Part model, mm, in its own coordinate system. Face numbers are marked on the shaded views. A direction names the side the tool comes from. Coordinates: 2 decimals unless noted, no trailing zeros. Order: outer loops, then holes, each group sorted by start corner. A loop starts at its lowest first (then second) coordinate and runs counter-clockwise, first axis right, second up.
1) Tool access for the marked faces 4, 5, 6 and 7: list every direction of +Z, -Z, +X, -X, +Y, -Y with a clear straight run to the whole face (end or side of a thin tool).
2) Wall check: L1, parallel to Z at x = -22, y = -8; L2, parallel to X at y = -13.5, z = 18.5; L3, parallel to X at y = -8.75, z = 11. Give the ranges that are in metal, low to high.
3) Cut at C-C (y = -8.5). List the corners of the cut face in (x, z).
4) Cut at B-B (z = 23). List the corners of the cut face in (x, y), and give its area (3 significant figures).
5) Cut at A-A (x = -9). List the corners of the cut face in (y, z).
6) Pin check, flat tips, straight feed: pin 1 Ø2 at (x, y) = (17, -13) entering from -Z; pin 2 Ø1 at (x, y) = (-63, -13.5) entering from -Z; pin 3 Ø12 at (y, z) = (-11, 22.5) entering from -X. Stop position of each tip, or through.
7) Mould opens along Z. For the marked faces 1, 2 and 3 say: +Z half, -Z half, draft (parallel to the pull), parting line (faces both ways), or undercut.
8) Cut at D-D (z = 33.5). List the corners of the cut face in (x, y), and give its area (3 significant figures).
```python
from build123d import *

# Parameters (mm, degrees)
F1_DEPTH = 20


with BuildPart() as f1:
    # F0 (on Front) → F1 (new body)
    with BuildSketch(Plane.XZ):
        with BuildLine():
            ThreePointArc((79.969927, 8.602908), (65.940764, 27.690839), (43.535016, 20))
            ThreePointArc((43.535016, 20), (40.035238, 10.217898), (41.914734, 0))
            ThreePointArc((41.914734, 0), (64.379924, -10.904832), (79.969927, 8.602908))
        make_face()
        Polygon((51.786245, 21.173801), (69.39666, 20.270671), (73.97965, 3.243089), (59.201679, -6.377406), (45.4854, 4.704383), align=None, mode=Mode.SUBTRACT)
        with BuildLine():
            ThreePointArc((-40.33078, 20), (-39.357032, 15.679199), (-39.030073, 11.262118))
            ThreePointArc((-39.030073, 11.262118), (-39.583722, 5.525184), (-41.224234, 0))
            Line((-41.224234, 0), (41.914734, 0))
            ThreePointArc((41.914734, 0), (40.035238, 10.217898), (43.535016, 20))
            Line((43.535016, 20), (-40.33078, 20))
        make_face()
        with BuildLine():
            ThreePointArc((-39, 9.656477), (-37.828427, 12.484904), (-35, 13.656477))
            Line((-35, 13.656477), (35, 13.656477))
            ThreePointArc((35, 13.656477), (37.828427, 12.484904), (39, 9.656477))
            Line((39, 9.656477), (39, 7.656477))
            ThreePointArc((39, 7.656477), (37.828427, 4.828049), (35, 3.656477))
            Line((35, 3.656477), (-35, 3.656477))
            ThreePointArc((-35, 3.656477), (-37.828427, 4.828049), (-39, 7.656477))
            Line((-39, 7.656477), (-39, 9.656477))
        make_face(mode=Mode.SUBTRACT)
        with BuildLine():
            ThreePointArc((-41.224234, 0), (-39.583722, 5.525184), (-39.030073, 11.262118))
            ThreePointArc((-39.030073, 11.262118), (-39.357032, 15.679199), (-40.33078, 20))
            ThreePointArc((-40.33078, 20), (-99.000183, 12.600964), (-41.224234, 0))
        make_face()
        Polygon((-92.124084, 11.262118), (-80.577079, 31.262118), (-57.483068, 31.262118), (-45.936063, 11.262118), (-57.483068, -8.737882), (-80.577079, -8.737882), align=None, mode=Mode.SUBTRACT)
    extrude(amount=F1_DEPTH)


solid = f1.part
```
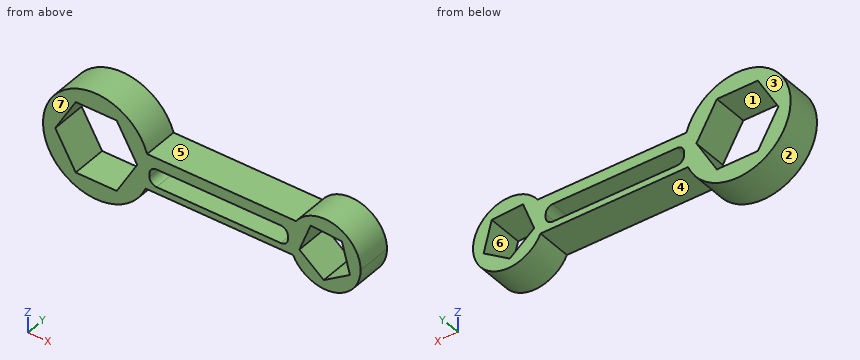
Geometry check:
1. face 4: -Z, +Y, -Y
1. face 5: +Z, +Y, -Y
1. face 6: +Y, -Y
1. face 7: +Z, -Z, +X, -X, -Y
2. L1: z = 0 to 3.66, 13.66 to 20
2. L2: x = -98.14 to -87.95, -50.11 to 50.76, 69.87 to 77.35
2. L3: x = -99.03 to -91.97, -46.09 to -38.77, 38.77 to 47.89, 71.89 to 79.83
3. outline: (-41.22, 0) - (41.91, 0) arc R20 ccw (long way) to (43.54, 20) - (-40.33, 20) arc R30 ccw (long way) to start; hole (-92.12, 11.26) - (-80.58, -8.74) - (-57.48, -8.74) - (-45.94, 11.26) - (-57.48, 31.26) - (-80.58, 31.26) - close; hole (-39, 7.66) arc R4 ccw to (-35, 3.66) - (35, 3.66) arc R4 ccw to (39, 7.66) - (39, 9.66) arc R4 ccw to (35, 13.66) - (-35, 13.66) arc R4 ccw to (-39, 9.66) - close; hole (45.49, 4.7) - (59.2, -6.38) - (73.98, 3.24) - (69.4, 20.27) - (51.79, 21.17) - close
4. outline: (-96.64, -20) - (-85.35, -20) - (-85.35, 0) - (-96.64, 0) - close; (-52.71, -20) - (-41.42, -20) - (-41.42, 0) - (-52.71, 0) - close; (46.09, -20) - (73.85, -20) - (73.85, 0) - (46.09, 0) - close
4. area: 1,010 mm2
5. outline: (-20, 0) - (0, 0) - (0, 3.66) - (-20, 3.66) - close; (-20, 13.66) - (0, 13.66) - (0, 20) - (-20, 20) - close
6. pin 1: stops at z = 0
6. pin 2: stops at z = -18.22
6. pin 3: stops at x = -98.57
7. face 1: undercut
7. face 2: parting line
7. face 3: draft
8. outline: (-89.17, -20) - (-48.89, -20) - (-48.89, 0) - (-89.17, 0) - close
8. area: 805 mm2
